from build123d import *

# Parameters (mm, degrees)
F0_R     = 2.75
F1_DEPTH = 5
F3_DEPTH = 6
F4_R     = 0.5
F5_DEPTH = 11.001


with BuildPart() as f1:
    # F0 (on Top) → F1 (new body)
    with BuildSketch(Plane.XY):
        Circle(F0_R)
    extrude(amount=-F1_DEPTH)

    # F2 (on Top) → F3 (join)
    with BuildSketch(Plane.XY):
        Polygon((1.732051, -3), (3.464102, 0), (1.732051, 3), (-1.732051, 3), (-3.464102, 0), (-1.732051, -3), align=None)
    extrude(amount=F3_DEPTH)

    # F4 (on face) → F5 (cut, through all)
    with BuildSketch(Plane.XY.offset(6)):
        Circle(F4_R)
    extrude(amount=-F5_DEPTH, mode=Mode.SUBTRACT)


solid = f1.part
Source: CAD feature listing. Evaluate the final solid. Frame: model axes, mm. A direction names the side the tool comes from. Give positions to 0.01 mm unless a question says otherwise; leave off trailing zeros. Write each loop counter-clockwise with the first axis right and the second up, starting at its lowest first coordinate (ties: lowest second). Pieces come first, ordered by that corner, then holes. Notation, with made-up numbers: (89, 61.25) -> (124, 61.25) arc R21 ccw to (124, 86.25) -> close; hole circle Ø9 at (25, 52). An arc over 180 degrees is marked (long way). Return JSON: item names as keys, results as strings. Group by question number.
1. Material intervals for line 1 (Y direction, x = 0, z = 1.5); line 2 (Z direction, x = 1.25, y = -2.5); line 3 (X direction, y = 2.5, z = -3.25), sorted ascending. Write a range as from..to.
2. Access query for faces 1 (the face through (-0.596, -2.685, -2.465)), 2 (the face through (-0.108, -0.488, 0.577)). Directions: +Z, -Z, +X, -X, +Y, -Y. A direction counts if a zero-diameter tool reaches every point of the face in a straight line with its end or side. Return the directions, or none.
3. Section D-D, the plane y = 1. Output: boundary loops of the cut face in (x, z).
4. Section B-B, the plane z = 2. Output: boundary loops of the cut face in (x, y), then the cut area to 3 significant figures.
5. Section A-A, the plane x = 0. Output: boundary loops of the cut face in (y, z).
6. Pin query (flat end, axial travel): pin 1 Ø1 at (x, z) = (-2.5, 1) entering from -Y. Return the tip coordinate at first contact, or that it passes through.
7. Section C-C, the plane y = -0.25. Output: boundary loops of the cut face in (x, z).
Determined:
{
 "1": {"line 1": "y = -3..-0.5, 0.5..3", "line 2": "z = 0..6", "line 3": "x = -1.15..1.15"},
 "2": {"face 1": "-Z", "face 2": "+Z, -Z"},
 "3": {"outline": "(-2.89, 0) -> (-2.56, 0) -> (-2.56, -5) -> (2.56, -5) -> (2.56, 0) -> (2.89, 0) -> (2.89, 6) -> (-2.89, 6) -> close"},
 "4": {"outline": "(-3.46, 0) -> (-1.73, -3) -> (1.73, -3) -> (3.46, 0) -> (1.73, 3) -> (-1.73, 3) -> close; hole circle Ø1 at (0, 0)", "area": "30.4 mm2"},
 "5": {"outline": "(-3, 0) -> (-2.75, 0) -> (-2.75, -5) -> (-0.5, -5) -> (-0.5, 6) -> (-3, 6) -> close; (0.5, -5) -> (2.75, -5) -> (2.75, 0) -> (3, 0) -> (3, 6) -> (0.5, 6) -> close"},
 "6": {"pin 1": "stops at y = -2.54"},
 "7": {"outline": "(-3.32, 0) -> (-2.74, 0) -> (-2.74, -5) -> (-0.43, -5) -> (-0.43, 6) -> (-3.32, 6) -> close; (0.43, -5) -> (2.74, -5) -> (2.74, 0) -> (3.32, 0) -> (3.32, 6) -> (0.43, 6) -> close"}
}
